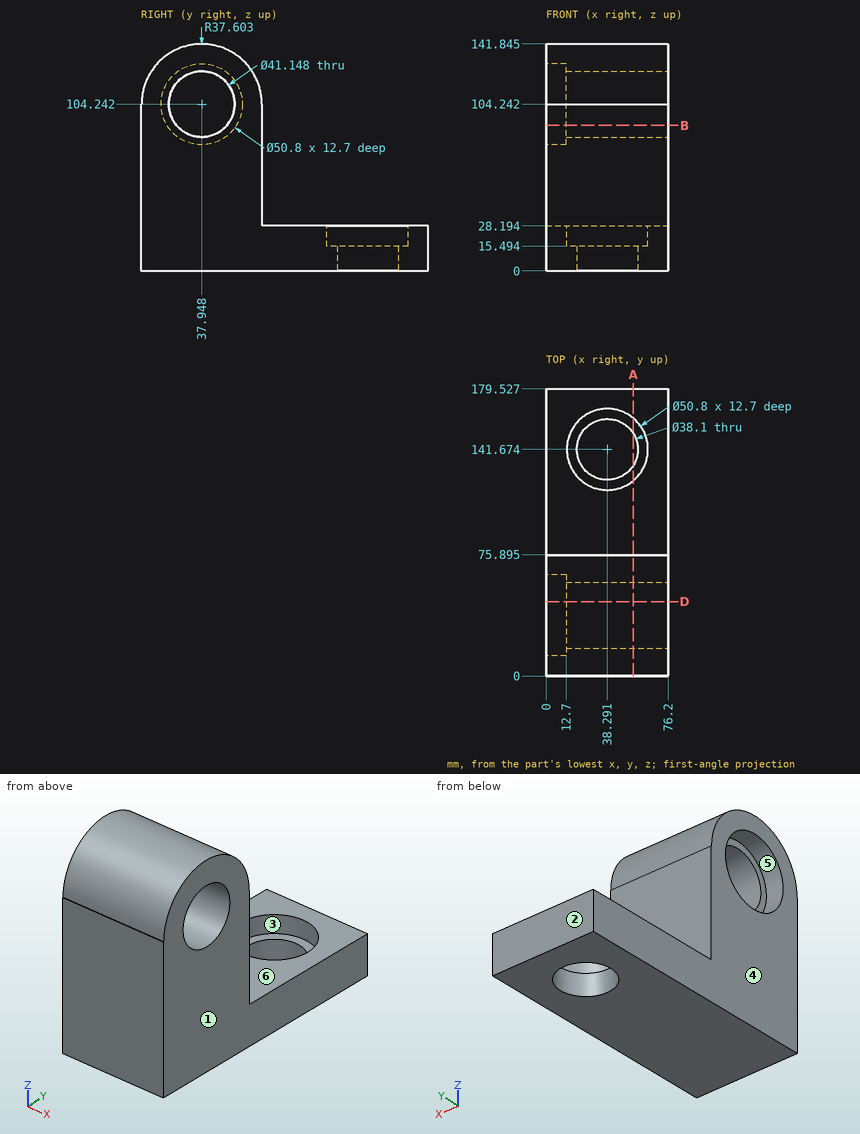
Job drawing, mm, ordinate dimensions from the low corner. One solid piece. A direction names the side the tool comes from. Coordinates: 2 decimals unless noted, no trailing zeros. Order: outer loops, then holes, each group sorted by start corner. A loop starts at its lowest first (then second) coordinate and runs counter-clockwise, first axis right, second up. Notation, with made-up numbers: (6.25, 79) - (64.25, 79) arc R6 cw to (64.25, 89) - close; hole circle Ø7 at (20.5, -19). An arc over 180 degrees is marked (long way). Use CSV: the item, a comma, the result in double quotes.
Item 1: Saw through at A-A on x = 54.5. Give the number of separate pieces and of enclosed holes in the cut face, and give its area (3 significant figures).
Solved:
separate pieces,"2"
enclosed holes,"1"
area,"10,900 mm²"
Item 2: Mould opens along X. For the marked faces 1, 2 and 3 say: +X half, -X half, draft (parallel to the pull), parting line (faces both ways), or undercut.
Solved:
face 1,"+X half"
face 2,"draft"
face 3,"undercut"
Item 3: Saw through at D-D on y = 46.5. Give the cut face in (x, z) (1 decimal).
Solved:
outline,"(0, 0) - (76.2, 0) - (76.2, 85.5) - (12.7, 85.5) - (12.7, 80.3) - (0, 80.3) - close; (0, 128.2) - (12.7, 128.2) - (12.7, 123) - (76.2, 123) - (76.2, 140.9) - (0, 140.9) - close"
Item 4: 3-axis set-ups, long thin cutter, end or side, ignore diameter. For the marked faces 4, 5 and 6: which of +Z, -Z, +X, -X, +Y, -Y reach the whole face in a straight line?
Solved:
face 4,"+Z, -Z, -X, +Y, -Y"
face 5,"-X"
face 6,"+Z, +X, -X, +Y"
Item 5: Saw through at B-B on z = 91. Give the cut face in (x, y) (1 decimal).
Solved:
outline,"(0, 0) - (76.2, 0) - (76.2, 22.2) - (12.7, 22.2) - (12.7, 16.3) - (0, 16.3) - close; (0, 59.6) - (12.7, 59.6) - (12.7, 53.7) - (76.2, 53.7) - (76.2, 75.9) - (0, 75.9) - close"
Item 6: Drop flat-ended pins along their axis: P1, Ø10, axis at x = 29, z = 78, coming from the -Y side; P2, Ø1.5, axis at x = 54.5, y = 34.5, coming from the +Z side; P3, Ø6, axis at x = 62.5, z = 50.5, coming from the +Y side (1 decimal); P4, Ø1, axis at x = 58.5, z = 122, coming from the -Y side. Give the stop position or say it passes through.
Solved:
P1,"stops at y = 0"
P2,"stops at z = 141.75"
P3,"stops at y = 75.9"
P4,"stops at y = 4.54"
Item 7: Probe probe 1 along Z at (x, y) = (70, 154.5) (1 decimal); probe 2 along Y at (x, z) = (71.5, 104) (1 decimal); probe 3 along Y at (x, z) = (42, 116) (1 decimal). List the from-to ranges inside material, lowest first.
Solved:
probe 1,"z = 0 to 28.2"
probe 2,"y = 0 to 17.4, 58.5 to 75.9"
probe 3,"y = 2.2 to 21.1, 54.8 to 73.7"
